from build123d import *

# Parameters (mm, degrees)
F0_R      = 2
F1_DEPTH  = 25
F3_DEPTH  = 276
F4_R      = 2
F5_DEPTH  = 84.8
F6_R      = 2.5
F7_DEPTH  = 5
F9_DEPTH  = 20
F10_R     = 2
F11_DEPTH = 25
F14_DEPTH = 2


with BuildPart() as f1:
    # F0 (on Top) → F1 (new body)
    with BuildSketch(Plane.XY):
        with BuildLine():
            Line((-51.434658, 66.572686), (-81.434658, 66.572686))
            Line((-81.434658, 66.572686), (-81.434658, -43.427314))
            Line((-81.434658, -43.427314), (-6.434658, -43.427314))
            ThreePointArc((-6.434658, -43.427314), (8.565342, -58.427314), (23.565342, -43.427314))
            Line((23.565342, -43.427314), (98.565342, -43.427314))
            Line((98.565342, -43.427314), (98.565342, 66.572686))
            Line((98.565342, 66.572686), (68.565342, 66.572686))
            ThreePointArc((68.565342, 66.572686), (53.565342, 81.572686), (38.565342, 66.572686))
            Line((38.565342, 66.572686), (-21.434658, 66.572686))
            ThreePointArc((-21.434658, 66.572686), (-36.434658, 81.572686), (-51.434658, 66.572686))
        make_face()
        with Locations((8.565342, -50.927314)):
            Circle(F0_R, mode=Mode.SUBTRACT)
        with Locations((-36.434658, 74.072686)):
            Circle(F0_R, mode=Mode.SUBTRACT)
        with Locations((53.565342, 74.072686)):
            Circle(F0_R, mode=Mode.SUBTRACT)
    extrude(amount=F1_DEPTH)

    # F2 (on face) → F3 (cut)
    with BuildSketch(Plane.YZ.offset(98.565342)):
        with BuildLine():
            Line((43.145373, 0), (22.822686, 0))
            ThreePointArc((22.822686, 0), (11.572686, 11.25), (0.322686, 0))
            Line((0.322686, 0), (-20, 0))
            ThreePointArc((-20, 0), (-41.231841, 11.150842), (-64.902842, 15))
            Line((-64.902842, 15), (-64.902842, -16.413443))
            Line((-64.902842, -16.413443), (88.048215, -16.413443))
            Line((88.048215, -16.413443), (88.048215, 15))
            ThreePointArc((88.048215, 15), (64.377213, 11.150842), (43.145373, 0))
        make_face()
    extrude(amount=-F3_DEPTH, mode=Mode.SUBTRACT)

    # F4 (on face) → F5 (cut)
    with BuildSketch(Plane.XY.offset(25)):
        with Locations((-56.434658, 32.872686)):
            Circle(F4_R)
        with Locations((73.565342, 32.872686)):
            Circle(F4_R)
        with Locations((-56.434658, -9.727314)):
            Circle(F4_R)
        with Locations((73.565342, -9.727314)):
            Circle(F4_R)
    extrude(amount=-F5_DEPTH, mode=Mode.SUBTRACT)

    # F6 (on face) → F7 (cut)
    with BuildSketch(Plane.XY.offset(25)):
        with Locations((-56.434658, 32.872686)):
            Circle(F6_R)
        with Locations((73.565342, 32.872686)):
            Circle(F6_R)
        with Locations((73.565342, -9.727314)):
            Circle(F6_R)
        with Locations((-56.434658, -9.727314)):
            Circle(F6_R)
    extrude(amount=-F7_DEPTH, mode=Mode.SUBTRACT)


with BuildPart() as f9:
    # F8 (on face) → F9 (new body)
    with BuildSketch(Plane(origin=(-81.434658, 0, 0), x_dir=(0, -1, 0), z_dir=(-1, 0, 0))):
        with BuildLine():
            ThreePointArc((-0.322686, 0), (-11.572686, -11.25), (-22.822686, 0))
            Line((-22.822686, 0), (-43.145373, 0))
            ThreePointArc((-43.145373, 0), (-41.680906, -3.535534), (-38.145373, -5))
            Line((-38.145373, -5), (-30.322686, -5))
            ThreePointArc((-30.322686, -5), (-27.750207, -5.712535), (-25.910922, -7.647059))
            ThreePointArc((-25.910922, -7.647059), (-11.572686, -16.25), (2.765549, -7.647059))
            ThreePointArc((2.765549, -7.647059), (4.604835, -5.712535), (7.177314, -5))
            Line((7.177314, -5), (15, -5))
            ThreePointArc((15, -5), (18.535534, -3.535534), (20, 0))
            Line((20, 0), (-0.322686, 0))
        make_face()
    extrude(amount=F9_DEPTH)

    # F10 (on face) → F11 (cut)
    with BuildSketch(Plane.XY):
        with Locations((-91.434658, 32.984029)):
            Circle(F10_R)
        with Locations((-91.434658, -10.871857)):
            Circle(F10_R)
    extrude(amount=-F11_DEPTH, mode=Mode.SUBTRACT)

    # F13 (on face) + F12 (on face) → F14 (cut)
    with BuildSketch(Plane(origin=(0, 0, -5), x_dir=(1, 0, 0), z_dir=(0, 0, -1))):
        Polygon((-89.965689, 8.371431), (-88.534741, 10.893809), (-90.00371, 13.394235), (-92.903627, 13.372283), (-94.334575, 10.849906), (-92.865606, 8.34948), align=None)
    with BuildSketch(Plane(origin=(0, 0, -5), x_dir=(1, 0, 0), z_dir=(0, 0, -1))):
        Polygon((-89.982201, -35.494083), (-88.534659, -32.981191), (-89.987117, -30.471138), (-92.887115, -30.473976), (-94.334657, -32.986868), (-92.882199, -35.496921), align=None)
    extrude(amount=-F14_DEPTH, mode=Mode.SUBTRACT)


solid = f9.part
Check sheet for the modelled part. Datum: model origin and axes. Units: mm. A direction names the side the tool comes from. Round coordinates to 2 decimals unless told otherwise and drop trailing zeros. Loops run counter-clockwise (first coordinate to the right, second up) from the corner with the lowest first, then second, coordinate; pieces in that order, holes last. Notation, with made-up numbers: (-21, 58.5) -> (35, 58.5) arc R23 cw to (35, 67.5) -> close; hole circle Ø4 at (28, -12.75). An arc over 180 degrees is marked (long way). Put each result on its own line as item: value. Start each with the question number.
1. Section check C-C (z = -1.5). Enter the section's corners in (x, y), plus the area to 3 significant figures.
2. Section check A-A (z = -6.5). Enter the section's corners in (x, y), plus the area to 3 significant figures.
3. Section check D-D (x = -91.25). Enter the section's corners in (y, z), plus the area to 3 significant figures.
4. Access from +Z, -Z, +X, -X, +Y, -Y to the whole of each face (thin tool, end or side, straight path). Record for faces 4 (the face through (-89.26, -12.13, -4.01)), 5 (the face through (-89.527, 33.585, -1.479)).
5. Scan lines: probe 1 along Y at (x, z) = (-96, -2.75); probe 2 along Y at (x, z) = (-83.25, -5.5); probe 3 along X at (y, z) = (-10.5, -3.25). Record each from-to range of solid material in increasing order.
6. Gauge pin test, flat ends, axial feed: pin 1 (1 mm diameter, centred on x = -86.5, y = 13.5, fed in from -Z); pin 2 (6 mm diameter, centred on x = -97, y = 9, fed in from +Z); pin 3 (8.5 mm diameter, centred on x = -88.5, y = -13, fed in from -Z); pin 4 (6 mm diameter, centred on x = -84, z = -3, fed in from +Y). Record the tip position at first contact, or that the pin passes through.
7. Section check B-B (x = -96.75). Enter the section's corners in (y, z), plus the area to 3 significant figures.
8. Draft check along Y on faces 1 (the face through (-91.295, -4.572, -5.732)), 2 (the face through (-89.9, 34.5, -3)), 3 (the face through (-81.435, 12, -12)). Enter one of: +Y half, -Y half, draft (parallel to the pull), parting line (faces both ways), or undercut.
Findings:
1. outline: (-101.43, -19.77) -> (-81.43, -19.77) -> (-81.43, 0.42) -> (-101.43, 0.42) -> close; (-101.43, 22.72) -> (-81.43, 22.72) -> (-81.43, 42.92) -> (-101.43, 42.92) -> close; hole circle Ø4 at (-91.43, -10.87); hole circle Ø4 at (-91.43, 32.98)
1. area: 783 mm^2
2. outline: (-101.43, -3.61) -> (-81.43, -3.61) -> (-81.43, 2.39) -> (-101.43, 2.39) -> close; (-101.43, 20.75) -> (-81.43, 20.75) -> (-81.43, 26.75) -> (-101.43, 26.75) -> close
2. area: 240 mm^2
3. outline: (-20, 0) arc R5 ccw to (-15, -5) -> (-13.38, -5) -> (-13.38, -3) -> (-12.86, -3) -> (-12.86, 0) -> close; (-8.88, -3) -> (-8.36, -3) -> (-8.36, -5) -> (-7.18, -5) arc R5 cw to (-2.77, -7.65) arc R16.25 ccw to (25.91, -7.65) arc R5 cw to (30.32, -5) -> (30.47, -5) -> (30.47, -3) -> (30.99, -3) -> (30.99, 0) -> (22.82, 0) arc R11.25 cw to (0.32, 0) -> (-8.88, 0) -> close; (34.98, -3) -> (35.5, -3) -> (35.5, -5) -> (38.15, -5) arc R5 ccw to (43.15, 0) -> (34.98, 0) -> close
3. area: 321 mm^2
4. face 4: -Z
4. face 5: +Z, -Z
5. probe 1: y = -19.18 to 0.66, 22.48 to 42.32
5. probe 2: y = -5 to 1.76, 21.39 to 28.14
5. probe 3: x = -101.43 to -94.13, -88.76 to -81.43
6. pin 1: stops at z = -16.19
6. pin 2: stops at z = -9.77
6. pin 3: stops at z = -5
6. pin 4: stops at y = 43.15
7. outline: (-20, 0) arc R5 ccw to (-15, -5) -> (-7.18, -5) arc R5 cw to (-2.77, -7.65) arc R16.25 ccw to (25.91, -7.65) arc R5 cw to (30.32, -5) -> (38.15, -5) arc R5 ccw to (43.15, 0) -> (22.82, 0) arc R11.25 cw to (0.32, 0) -> close
7. area: 365 mm^2
8. face 1: -Y half
8. face 2: undercut
8. face 3: draft
